from build123d import *

# Parameters (mm, degrees)
SKETCH2_R               = 5.2324
SKETCH1_R               = 5.8801
DOME1_FACE_RADIUS       = 5.2324
DOME1_HEIGHT            = 14.986
CUT_EXTRUDE1_DEPTH      = 19.644941044
CUT_EXTRUDE1_DEPTH_BACK = 19.644941044
SKETCH3_R               = 1.5494
SKETCH4_R               = 2.2225
CUT_EXTRUDE2_DEPTH      = 14.1732


with BuildPart() as part:
    # Sketch2 → Loft1 section 0
    with BuildSketch(Plane.XY.offset(1.7018)):
        Circle(SKETCH2_R)
    # Sketch1 → Loft1 section 1
    with BuildSketch(Plane.XY):
        Circle(SKETCH1_R)
    loft()

    # Dome1: an elliptical dome of height H over a round flat face of radius A is half a spheroid: the quarter ellipse of half axes A and H revolved about the face's axis
    with BuildSketch(Plane((0, 0, 1.7018), x_dir=(0, 1, 0), z_dir=(1, 0, 0)), mode=Mode.PRIVATE) as dome1_quarter:
        Ellipse(DOME1_FACE_RADIUS, DOME1_HEIGHT)
        Rectangle(DOME1_FACE_RADIUS, DOME1_HEIGHT, align=(Align.MIN, Align.MIN), mode=Mode.INTERSECT)
    revolve(dome1_quarter.sketch, axis=Axis((0, 0, 1.7018), (0, 0, 1)))

    # Sketch3 → Cut-Extrude1 (cut, two sides: drawn at the far end of the back side and taken through both)
    with BuildSketch(Plane(origin=(0, 0, 0), x_dir=(1, 0, 0), z_dir=(0, 1, 0)).offset(-CUT_EXTRUDE1_DEPTH_BACK)):
        with Locations(Location((0, -11.0998, 0), (0, 0, 270))):
            Circle(SKETCH3_R)
    extrude(amount=CUT_EXTRUDE1_DEPTH + CUT_EXTRUDE1_DEPTH_BACK, mode=Mode.SUBTRACT)

    # Sketch4 → Cut-Extrude2 (cut)
    with BuildSketch(Plane(origin=(0, 0, 0), x_dir=(-1, 0, 0), z_dir=(0, 0, -1))):
        Circle(SKETCH4_R)
    extrude(amount=-CUT_EXTRUDE2_DEPTH, mode=Mode.SUBTRACT)


solid = part.part
Build history of the part. All positions in model axes, mm. A direction names the side the tool comes from. Coordinates: 2 decimals unless noted, no trailing zeros. Use CSV: the item, a comma, the result in double quotes. Start each with the question number.
Q1. Flat gauge pins, fed straight in: pin 1 Ø3 at (x, z) = (0, 11.1) entering from +Y; pin 2 Ø3 at (x, z) = (-2, 13.5) entering from -Y; pin 3 Ø3 at (x, y) = (-2.5, -4) entering from -Z; pin 4 Ø1 at (y, z) = (0, 10) entering from -X. Where does each tip first touch, or does it go through?
Q2. Cut at A-A, the plane x = -0.25. State how many separate pieces and enclosed holes the cut face has, then the cut area to 3 significant figures.
Q3. Pull direction X, two halves, no side cores. Call faces 1 (the flat face through (3, 0, 0)), 2 (the cylindrical face through (2.22, 0.1, 6.99)), 3 (the cylindrical face through (0.07, 3.01, 9.55)): released by +X, released by -X, zero draft, split by the parting line, or undercut.
Q4. 3-axis set-ups, long thin cutter, end or side, ignore diameter. For faces 4 (the cylindrical face through (0.07, -3.05, 9.55)), 5 (the flat face through (0, 0, 14.173)): which of +Z, -Z, +X, -X, +Y, -Y reach the whole face in a straight line?
Q5. Drill centre lines: probe 1 along Z at (x, y) = (0, 3.8); probe 2 along Y at (x, z) = (1, 8.5); probe 3 along Y at (x, z) = (-1.75, 9.75). Where is each one in solid material? Low to high.
Checked values:
1,pin 1,"passes through"
1,pin 2,"stops at y = -3.53"
1,pin 3,"stops at z = 0"
1,pin 4,"stops at x = -4.47"
2,separate pieces,"3"
2,enclosed holes,"0"
2,area,"67.9 mm²"
3,face 1,"zero draft"
3,face 2,"undercut"
3,face 3,"undercut"
4,face 4,"+Y, -Y"
4,face 5,"-Z"
5,probe 1,"z = 0 to 9.55"
5,probe 2,"y = -4.55 to -1.98, 1.98 to 4.55"
5,probe 3,"y = -4.05 to -1.37, 1.37 to 4.05"
